CAD build for the part. Positions are in the model's coordinates, mm. A direction names the side the tool comes from. Round coordinates to 2 decimals unless told otherwise and drop trailing zeros. Write each loop counter-clockwise with the first axis right and the second up, starting at its lowest first coordinate (ties: lowest second). Pieces come first, ordered by that corner, then holes. Notation, with made-up numbers: (73, 85.5) - (108, 85.5) arc R15 cw to (108, 91.5) - close; hole circle Ø1 at (13.25, 23.5). An arc over 180 degrees is marked (long way). Answer in a Markdown table with one row per item.
```python
from build123d import *

# Parameters (mm, degrees)
F0_R     = 2.865
F1_DEPTH = 19.88
F3_R     = 1.44
F4_DEPTH = 50
F5_R     = 2.675
F5_R_2   = 1.44
F6_DEPTH = 3.06


with BuildPart() as f1:
    # F0 (on Top) → F1 (new body)
    with BuildSketch(Plane.XY):
        Circle(F0_R)
    extrude(amount=F1_DEPTH)

    # F3 (on Front) → F4 (join)
    with BuildSketch(Plane.XZ):
        with Locations((0, 9.94)):
            Circle(F3_R)
    extrude(amount=-F4_DEPTH)

    # F5 (on face) → F6 (join)
    with BuildSketch(Plane(origin=(0, 50, 0), x_dir=(-1, 0, 0), z_dir=(0, 1, 0))):
        with Locations((0, 9.94)):
            Circle(F5_R)
        with Locations((0, 9.94)):
            Circle(F5_R_2, mode=Mode.SUBTRACT)
    extrude(amount=-F6_DEPTH)


solid = f1.part
```
Q1. Saw through at C-C on y = 45.5. List the corners of the cut face in (x, z).
Computed:
| item | result |
|---|---|
| outline | circle Ø2.88 at (0, 9.94) |
Q2. Saw through at B-B on z = 9.94. List the corners of the cut face in (x, y) (3 decimals).
Computed:
| item | result |
|---|---|
| outline | (-2.675, 46.94) - (-1.44, 46.94) - (-1.44, 2.477) arc R2.865 ccw (long way) to (1.44, 2.477) - (1.44, 46.94) - (2.675, 46.94) - (2.675, 50) - (-2.675, 50) - close |
Q3. 3-axis set-ups, long thin cutter, end or side, ignore diameter. For faces 1 (the flat face through (-1.2, 46.94, 8.8)), 2 (the flat face through (0, 0, 19.88)), 3 (the cylindrical face through (0.3, 48.5, 12.6)): which of +Z, -Z, +X, -X, +Y, -Y reach the whole face in a straight line?
Computed:
| item | result |
|---|---|
| face 1 | none |
| face 2 | +Z, +X, -X, +Y, -Y |
| face 3 | +Y |
Q4. Saw through at A-A on x = 0. List the corners of the cut face in (y, z) (3 decimals).
Computed:
| item | result |
|---|---|
| outline | (-2.865, 0) - (2.865, 0) - (2.865, 8.5) - (46.94, 8.5) - (46.94, 7.265) - (50, 7.265) - (50, 12.615) - (46.94, 12.615) - (46.94, 11.38) - (2.865, 11.38) - (2.865, 19.88) - (-2.865, 19.88) - close |
Q5. Pull direction Y, two halves, no side cores. Call faces 4 (the cylindrical face through (-0.312, 24.397, 8.534)), 5 (the flat face through (0, 50, 10)), 6 (the flat face through (0, 0, 0)): released by +Y, released by -Y, zero draft, split by the parting line, or undercut.
Computed:
| item | result |
|---|---|
| face 4 | undercut |
| face 5 | released by +Y |
| face 6 | zero draft |
Q6. Drill centre lines: line 1 (Y direction, x = 1, z = 12); line 2 (Y direction, x = -1.55, z = 8.75); line 3 (Z direction, x = -1.3, y = 8.5). Where is each one in solid material? Low to high.
Computed:
| item | result |
|---|---|
| line 1 | y = -2.68 to 2.68, 46.94 to 50 |
| line 2 | y = -2.41 to 2.41, 46.94 to 50 |
| line 3 | z = 9.32 to 10.56 |
Q7. Flat gauge pins, fed straight in: pin 1 (1.6 mm diameter, centred on x = -1, z = 10, fed in from -Y); pin 2 (1 mm diameter, centred on x = 1.5, z = 4, fed in from -Y); pin 3 (3 mm diameter, centred on y = 26, z = 14.5, fed in from -X); pin 4 (3 mm diameter, centred on x = 0, y = 41.5, fed in from -Z). Where does each tip first touch, or does it go through?
Computed:
| item | result |
|---|---|
| pin 1 | stops at y = -2.86 |
| pin 2 | stops at y = -2.68 |
| pin 3 | passes through |
| pin 4 | stops at z = 8.5 |
Q8. Saw through at D-D on z = 14.25. List the corners of the cut face in (x, y) (3 decimals).
Computed:
| item | result |
|---|---|
| outline | circle Ø5.73 at (0, 0) |
